Drawing for the job (mm, zero at the part's lowest x, y, z). Round coordinates to 2 decimals unless told otherwise and drop trailing zeros. Write each loop counter-clockwise with the first axis right and the second up, starting at its lowest first coordinate (ties: lowest second). Pieces come first, ordered by that corner, then holes.
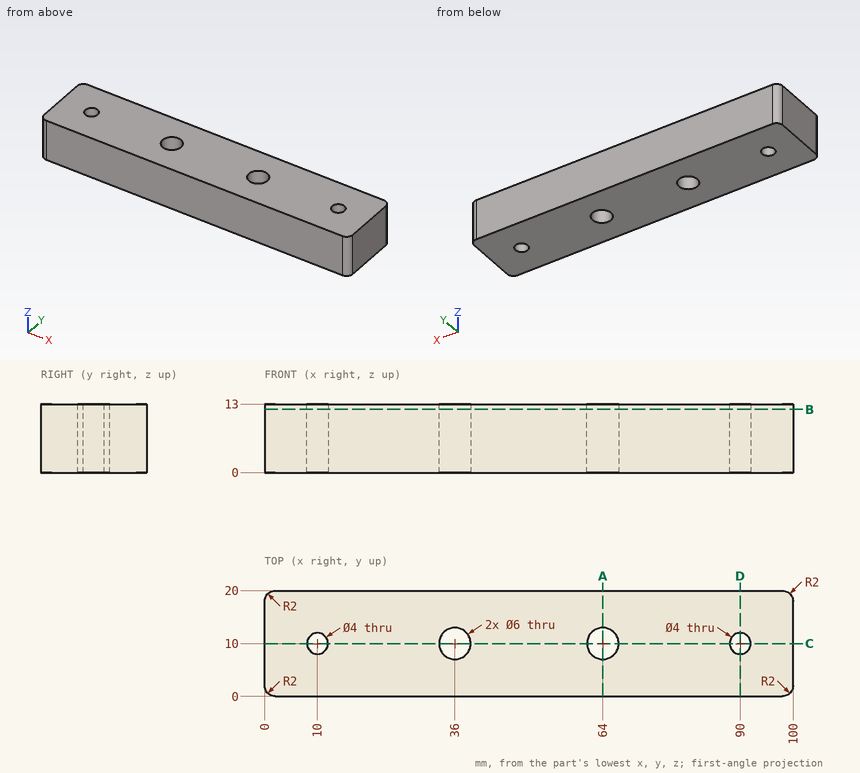
1) Cut at B-B on z = 12. List the corners of the cut face in (x, y).
2) Cut at C-C on y = 10. List the corners of the cut face in (x, z), and give its area (3 significant figures).
3) Cut at A-A on x = 64. List the corners of the cut face in (y, z), and give its area (3 significant figures).
4) Cut at D-D on x = 90. List the corners of the cut face in (y, z), and give its area (3 significant figures).
5) Wall check: probe 1 along X at (y, z) = (10.25, 6.5); probe 2 along Y at (x, z) = (36, 10); probe 3 along Y at (x, z) = (10, 3.75). Give the ranges that are in metal, low to high.
Result sheet:
1. outline: (0, 2) arc R2 ccw to (2, 0) - (98, 0) arc R2 ccw to (100, 2) - (100, 18) arc R2 ccw to (98, 20) - (2, 20) arc R2 ccw to (0, 18) - close; hole circle Ø4 at (10, 10); hole circle Ø6 at (36, 10); hole circle Ø6 at (64, 10); hole circle Ø4 at (90, 10)
2. outline: (0, 0) - (8, 0) - (8, 13) - (0, 13) - close; (12, 0) - (33, 0) - (33, 13) - (12, 13) - close; (39, 0) - (61, 0) - (61, 13) - (39, 13) - close; (67, 0) - (88, 0) - (88, 13) - (67, 13) - close; (92, 0) - (100, 0) - (100, 13) - (92, 13) - close
2. area: 1,040 mm2
3. outline: (0, 0) - (7, 0) - (7, 13) - (0, 13) - close; (13, 0) - (20, 0) - (20, 13) - (13, 13) - close
3. area: 182 mm2
4. outline: (0, 0) - (8, 0) - (8, 13) - (0, 13) - close; (12, 0) - (20, 0) - (20, 13) - (12, 13) - close
4. area: 208 mm2
5. probe 1: x = 0 to 8.02, 11.98 to 33.01, 38.99 to 61.01, 66.99 to 88.02, 91.98 to 100
5. probe 2: y = 0 to 7, 13 to 20
5. probe 3: y = 0 to 8, 12 to 20
